The model under review builds one solid part; all positions refer to its coordinate system, in mm. Face numbers are marked on the shaded views. A direction names the side the tool comes from. Round coordinates to 2 decimals unless told otherwise and drop trailing zeros. Write each loop counter-clockwise with the first axis right and the second up, starting at its lowest first coordinate (ties: lowest second). Pieces come first, ordered by that corner, then holes. Notation, with made-up numbers: (38, 80) -> (55, 80) arc R25 ccw to (55, 98) -> close; hole circle Ø3 at (-20, 21). An arc over 180 degrees is marked (long way). Use CSV: the item, a comma, the result in double quotes. Start each with the question number.
1) Take a section at C-C, the plane z = 40. State how many separate pieces and enclosed holes the cut face has, then the cut area to 3 significant figures.
2) For pin 1 Ø1 at (y, z) = (17.5, 13) entering from -X; pin 2 Ø16 at (y, z) = (30.5, 34) entering from -X; pin 3 Ø9.5 at (x, y) = (60.5, 25) entering from +Z, all flat-tipped, find the tip position at first contact; note any pin that passes through.
3) Mouldability with a two-part tool opening along Y and no side actions: class the marked faces 4, 5, 6 and 7 as released by +Y, released by -Y, zero draft, split by the parting line, or undercut.
4) Wall thickness on probe 1 along X at (y, z) = (2.5, 77); probe 2 along Y at (x, z) = (11.5, 73.5); probe 3 along Y at (x, z) = (58.25, 39.4): over which ranges is each line inside the solid? List them lowest first. Write a range as [from, to].
5) Take a section at D-D, the plane z = 71. Give the boundary of the cut face in (x, y).
6) Take a section at A-A, the plane x = 4. Give the boundary of the cut face in (y, z), then the cut area to 3 significant figures.
7) Machinability: for the marked faces 1, 2 and 3, which of the approach directions +Z, -Z, +X, -X, +Y, -Y give a long, thin tool a straight path to every point of the face, cutting with its end or side? Answer none if there is none.
8) Take a section at B-B, the plane y = 20. Give the boundary of the cut face in (x, z).
from build123d import *

# Parameters (mm, degrees)
BOSS_EXTRUDE1_DEPTH = 80
SKETCH2_R           = 2.1
BOSS_EXTRUDE2_DEPTH = 2
SKETCH3_W           = 3
SKETCH3_H           = 5
SKETCH3_H_2         = 7
BOSS_EXTRUDE3_DEPTH = 14.5
SKETCH5_W           = 3
SKETCH5_H           = 5
SKETCH5_H_2         = 7
BOSS_EXTRUDE4_DEPTH = 14.5
SKETCH8_R           = 2.5
CUT_EXTRUDE1_DEPTH  = 10


with BuildPart() as part:
    # Sketch1 → Boss-Extrude1 (new body)
    with BuildSketch(Plane.XY):
        Polygon((0, 0), (0, 50), (12, 50), (12, 52), (-2, 52), (-2, 25), (-2, -2), (50, -2), (50, 52), (36, 52), (36, 50), (48, 50), (48, 0), align=None)
    extrude(amount=BOSS_EXTRUDE1_DEPTH)

    # Sketch2 → Boss-Extrude2 (add)
    with BuildSketch(Plane.XZ.offset(2)):
        with BuildLine():
            Line((60, 45), (50, 45))
            Line((50, 45), (50, 35))
            Line((50, 35), (60, 35))
            ThreePointArc((60, 35), (65, 40), (60, 45))
        make_face()
        with Locations((60, 40)):
            Circle(SKETCH2_R, mode=Mode.SUBTRACT)
        with BuildLine():
            Line((-2, 35), (-2, 45))
            Line((-2, 45), (-12, 45))
            ThreePointArc((-12, 45), (-17, 40), (-12, 35))
            Line((-12, 35), (-2, 35))
        make_face()
        with Locations((-12, 40)):
            Circle(SKETCH2_R, mode=Mode.SUBTRACT)
    extrude(amount=-BOSS_EXTRUDE2_DEPTH)

    # Sketch3 → Boss-Extrude3 (add)
    with BuildSketch(Plane.ZY.offset(2)):
        with Locations((40, 27.5)):
            Rectangle(SKETCH3_W, SKETCH3_H)
        with Locations((40, 21.5)):
            Rectangle(SKETCH3_W, SKETCH3_H_2)
    extrude(amount=BOSS_EXTRUDE3_DEPTH)

    # Sketch5 → Boss-Extrude4 (add)
    with BuildSketch(Plane(origin=(50, 0, 0), x_dir=(0, 0, -1), z_dir=(1, 0, 0))):
        with Locations((-40, 27.5)):
            Rectangle(SKETCH5_W, SKETCH5_H)
        with Locations((-40, 21.5)):
            Rectangle(SKETCH5_W, SKETCH5_H_2)
    extrude(amount=BOSS_EXTRUDE4_DEPTH)

    # Sketch8 → Cut-Extrude1 (cut)
    with BuildSketch(Plane(origin=(0, 0, 38.5), x_dir=(-1, 0, 0), z_dir=(0, 0, -1))):
        with Locations((-58.25, 24)):
            Circle(SKETCH8_R)
        with Locations((10.25, 24)):
            Circle(SKETCH8_R)
    extrude(amount=-CUT_EXTRUDE1_DEPTH, mode=Mode.SUBTRACT)


solid = part.part
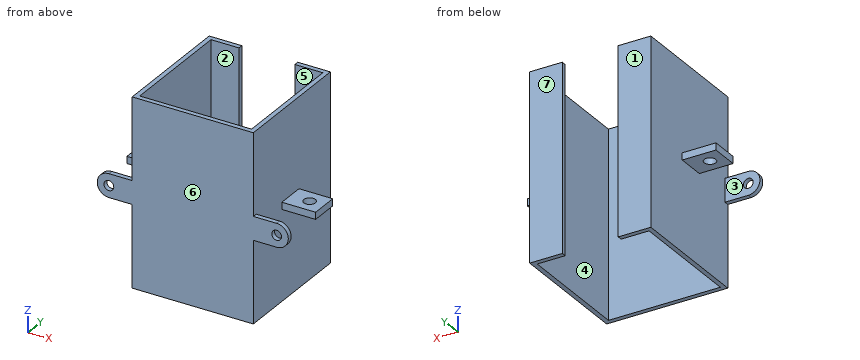
Values found:
1,separate pieces,"3"
1,enclosed holes,"2"
1,area,"712 mm²"
2,pin 1,"x = -2"
2,pin 2,"x = -16.5"
2,pin 3,"z = 41.5"
3,face 4,"undercut"
3,face 5,"undercut"
3,face 6,"released by -Y"
3,face 7,"released by +Y"
4,probe 1,"[-2, 0], [48, 50]"
4,probe 2,"[-2, 0], [50, 52]"
4,probe 3,"[18, 21.5], [26.5, 30]"
5,outline,"(-2, -2) -> (50, -2) -> (50, 52) -> (36, 52) -> (36, 50) -> (48, 50) -> (48, 0) -> (0, 0) -> (0, 50) -> (12, 50) -> (12, 52) -> (-2, 52) -> close"
6,outline,"(-2, 0) -> (0, 0) -> (0, 80) -> (-2, 80) -> close; (50, 0) -> (52, 0) -> (52, 80) -> (50, 80) -> close"
6,area,"320 mm²"
7,face 1,"+Z, -Z, +X, -X, +Y"
7,face 2,"+Z, -Z"
7,face 3,"+Z, -Z, -X"
8,outline,"(-16.5, 38.5) -> (-2, 38.5) -> (-2, 0) -> (0, 0) -> (0, 80) -> (-2, 80) -> (-2, 41.5) -> (-16.5, 41.5) -> close; (48, 0) -> (50, 0) -> (50, 38.5) -> (64.5, 38.5) -> (64.5, 41.5) -> (50, 41.5) -> (50, 80) -> (48, 80) -> close"
